Input: part model. Units: mm. Frame: model coordinates. Coordinates: 2 decimals unless noted, no trailing zeros. Write each loop counter-clockwise with the first axis right and the second up, starting at its lowest first coordinate (ties: lowest second). Pieces come first, ordered by that corner, then holes.
1) Section query A-A (y = -3.5). Output: boundary loops of the cut face in (x, z), then the cut area to 3 significant figures.
2) Line query: L1, parallel to X at y = -4.5, z = 260.5; L2, parallel to Y at x = 12.25, z = 43.5. Output: solid intervals per line, ascending.
3) Pin query (flat end, axial travel): pin 1 Ø12 at (x, y) = (9, -11) entering from +Z. Return the tip coordinate at first contact, or that it passes through.
4) Section query C-C (z = 191). Output: boundary loops of the cut face in (x, y), then the cut area to 3 significant figures.
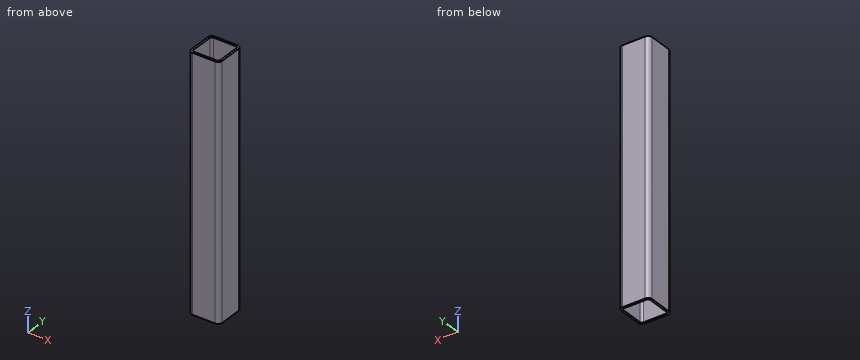
Autodesk Inventor part; units mm, degrees
ref_plane "Plano inicial" through (0, 0, 30) normal (0, 0, 1) x (1, 0, 0)
ref_plane "Plano final" through (0, 0, 275) normal (0, 0, 1) x (1, 0, 0)
ref_plane "Plano de trabalho4" through (218, 11, 30) normal (0, 0, -1) x (-1, 0, 0)
ref_plane "Plano inicial" through (0, 0, 30) normal (0, 0, 1) x (1, 0, 0)
ref_plane "Plano final" through (0, 0, 275) normal (0, 0, 1) x (1, 0, 0)
sketch "Esboço" plane through (0, 0, 0) normal (0, 0, 1) x (1, 0, 0)
  line L0 (-15, -11) -> (-15, 11)
  line L1 (-11, 15) -> (11, 15)
  line L2 (15, 11) -> (15, -11)
  line L3 (11, -15) -> (-11, -15)
  arc A0 (-15, -11) -> (-11, -15) centre (-11, -11) ccw
  arc A1 (15, 11) -> (11, 15) centre (11, 11) ccw
  arc A2 (-11, 15) -> (-15, 11) centre (-11, 11) ccw
  arc A3 (11, -15) -> (15, -11) centre (11, -11) ccw
  arc A4 (-11, 13) -> (-13, 11) centre (-11, 11) ccw
  line L4 (-11, 13) -> (11, 13)
  arc A5 (13, 11) -> (11, 13) centre (11, 11) ccw
  line L5 (13, 11) -> (13, -11)
  arc A6 (11, -13) -> (13, -11) centre (11, -11) ccw
  line L6 (11, -13) -> (-11, -13)
  arc A7 (-13, -11) -> (-11, -13) centre (-11, -11) ccw
  line L7 (-13, -11) -> (-13, 11)
  line L8 (0, 22.1598) -> (0, -22.1598) construction
  line L9 (-22.1598, 0) -> (22.1598, 0) construction
  dimension "d7" = 4
  dimension "d9" = 30
  dimension "d11" = 30
  dimension "d12" = 2
  dimension "d15" = 15
  dimension "d16" = 15
extrude "Corpo" add sketch "Esboço" along normal up to surface (245 mm away) from surface at 30
sketch "Sketch3" plane through (0, 0, 0) normal (0, 0, 1) x (1, 0, 0)
  line L0 (0, 0) -> (10, 0)
ref_plane "Work Plane3" through (0, 0, 0) normal (0, -1, 0) x (1, 0, 0)
sketch "Sketch4" plane through (0, 0, 0) normal (0, -1, 0) x (1, 0, 0)
  line L0 (-2, 30) -> (12, 30)
  line L1 (-2, 275) -> (12, 275)
  dimension "d18" = 245
ref_plane "Plano de trabalho4" through (218, 11, 30) normal (0, 0, -1) x (-1, 0, 0)
split "Dividir1" plane through (218, 11, 30) removes the side toward (0, 0, -1)
ref_plane "Plano de trabalho5" through (-332, 11, 275) normal (0, 0, 1) x (1, 0, 0)
split "Dividir2" plane through (-332, 11, 275) removes the side toward (0, 0, 1)
equation "\"d7\" = G_IR"
equation "\"d9\" = G_W"
equation "\"d11\" = G_H"
equation "\"d12\" = G_T"
equation "\"d15\" = 0.5 * d9"
equation "\"d16\" = 0.5 * d11"
equation "\"d3\" = G_L"
equation "\"G_W\" = 30"
equation "\"G_H\" = 30"
equation "\"G_T\" = 2"
equation "\"G_IR\" = 4"
equation "\"G_L\" = d18"
equation "\"G_OFFSET_END\" = 0"
equation "\"d14\" = G_OFFSET_END + B_L"
equation "\"B_L\" = 275"
properties part number "ISO 10799-2 - 30x30x2 - 245" material "Aço, suave"
Answer:
1. outline: (-15, 30) - (-13, 30) - (-13, 275) - (-15, 275) - close; (13, 30) - (15, 30) - (15, 275) - (13, 275) - close
1. area: 980 mm2
2. L1: x = -15 to -13, 13 to 15
2. L2: y = -14.8 to -12.56, 12.56 to 14.8
3. pin 1: stops at z = 275
4. outline: (-15, -11) arc R4 ccw to (-11, -15) - (11, -15) arc R4 ccw to (15, -11) - (15, 11) arc R4 ccw to (11, 15) - (-11, 15) arc R4 ccw to (-15, 11) - close; hole (-13, -11) arc R2 ccw to (-11, -13) - (11, -13) arc R2 ccw to (13, -11) - (13, 11) arc R2 ccw to (11, 13) - (-11, 13) arc R2 ccw to (-13, 11) - close
4. area: 214 mm2
